from build123d import *

# Parameters (mm, degrees)
SCHIZZO1_R                    = 18
ESTRUSIONE_ESTRUSIONE1_DEPTH  = 49.54
SCHIZZO2_R                    = 2.495
ESTRUSIONE_ESTRUSIONE2_DEPTH  = 2.5
SCHIZZO3_R                    = 1.575
ESTRUSIONE_ESTRUSIONE3_DEPTH  = 12.7
SCHIZZO4_R                    = 7.67
ESTRUSIONE_ESTRUSIONE4_DEPTH  = 5
SCHIZZO5_R                    = 4.01
ESTRUSIONE_ESTRUSIONE5_DEPTH  = 9.03
FORO_FILETTATO_M3X0_5_1_D     = 2.5
FORO_FILETTATO_M3X0_5_1_DEPTH = 9
FORO_FILETTATO_M3X0_5_1_TIP   = 0.751075774
ESTRUSIONE_ESTRUSIONE6_START  = -9.1
ESTRUSIONE_ESTRUSIONE6_DEPTH  = 9.1
ESTRUSIONE_ESTRUSIONE7_START  = -4.55
ESTRUSIONE_ESTRUSIONE7_DEPTH  = 3.4


with BuildPart() as part:
    # Schizzo1 → Estrusione-Estrusione1 (new body)
    with BuildSketch(Plane(origin=(0, 0, 0), x_dir=(0, 0, -1), z_dir=(1, 0, 0))):
        Circle(SCHIZZO1_R)
    extrude(amount=ESTRUSIONE_ESTRUSIONE1_DEPTH)

    # Schizzo2 → Estrusione-Estrusione2 (add)
    with BuildSketch(Plane.ZY):
        with Locations(Location((0, 0, 0), (0, 0, 180))):
            Circle(SCHIZZO2_R)
    extrude(amount=ESTRUSIONE_ESTRUSIONE2_DEPTH)

    # Schizzo3 → Estrusione-Estrusione3 (add)
    with BuildSketch(Plane.ZY.offset(2.5)):
        Circle(SCHIZZO3_R)
    extrude(amount=ESTRUSIONE_ESTRUSIONE3_DEPTH)

    # Schizzo4 → Estrusione-Estrusione4 (add)
    with BuildSketch(Plane.ZY.offset(13.72)):
        Circle(SCHIZZO4_R)
    extrude(amount=-ESTRUSIONE_ESTRUSIONE4_DEPTH)

    # Schizzo5 → Estrusione-Estrusione5 (add)
    with BuildSketch(Plane.ZY.offset(13.72)):
        Circle(SCHIZZO5_R)
    extrude(amount=-ESTRUSIONE_ESTRUSIONE5_DEPTH)

    # Foro filettato M3x0.5-1
    with Locations(Plane.ZY):
        with Locations((12.5, 0), (6.25, -10.825317547), (-6.25, -10.825317547), (-12.5, 0), (-6.25, 10.825317547), (6.25, 10.825317547)):
            Hole(FORO_FILETTATO_M3X0_5_1_D / 2, depth=FORO_FILETTATO_M3X0_5_1_DEPTH)
            with Locations((0, 0, -(FORO_FILETTATO_M3X0_5_1_DEPTH + FORO_FILETTATO_M3X0_5_1_TIP / 2))):  # 118° drill point
                Cone(0, FORO_FILETTATO_M3X0_5_1_D / 2, FORO_FILETTATO_M3X0_5_1_TIP, mode=Mode.SUBTRACT)

    # Schizzo10 → Estrusione-Estrusione6 (add)
    with BuildSketch(Plane(origin=(49.54, 0, 0), x_dir=(0, 0, -1), z_dir=(1, 0, 0)).offset(ESTRUSIONE_ESTRUSIONE6_START)):
        with BuildLine():
            ThreePointArc((-9.925, 15.016470124), (-5.181869246, 17.237988024), (0, 18))
            Line((0, 18), (0, 19.69938782))
            ThreePointArc((0, 19.69938782), (-4.26355498, 19.232472005), (-8.325, 17.85385828))
            ThreePointArc((-8.325, 17.85385828), (-9.134600688, 17.453508265), (-9.925, 17.016470124))
            Line((-9.925, 17.016470124), (-9.925, 15.016470124))
        make_face()
        with BuildLine():
            Line((0, 19.69938782), (0, 18))
            ThreePointArc((0, 18), (5.181869246, 17.237988024), (9.925, 15.016470124))
            Line((9.925, 15.016470124), (9.925, 17.016470124))
            ThreePointArc((9.925, 17.016470124), (9.134600688, 17.453508265), (8.325, 17.85385828))
            ThreePointArc((8.325, 17.85385828), (4.26355498, 19.232472005), (0, 19.69938782))
        make_face()
    extrude(amount=ESTRUSIONE_ESTRUSIONE6_DEPTH)

    # Schizzo10<4> → Estrusione-Estrusione7 (add, symmetric)
    with BuildSketch(Plane(origin=(49.54, 0, 0), x_dir=(0, 0, -1), z_dir=(1, 0, 0)).offset(ESTRUSIONE_ESTRUSIONE7_START)):
        with BuildLine():
            ThreePointArc((-8.325, 17.85385828), (-4.26355498, 19.232472005), (0, 19.69938782))
            Line((0, 19.69938782), (0, 21.990570068))
            ThreePointArc((0, 21.990570068), (-4.24218253, 21.577512815), (-8.325, 20.35385828))
            Line((-8.325, 20.35385828), (-8.325, 17.85385828))
        make_face()
        with BuildLine():
            Line((0, 21.990570068), (0, 19.69938782))
            ThreePointArc((0, 19.69938782), (4.26355498, 19.232472005), (8.325, 17.85385828))
            Line((8.325, 17.85385828), (8.325, 20.35385828))
            ThreePointArc((8.325, 20.35385828), (4.24218253, 21.577512815), (0, 21.990570068))
        make_face()
    extrude(amount=ESTRUSIONE_ESTRUSIONE7_DEPTH, both=True)


solid = part.part
Input: part model. Units: mm. Frame: model coordinates. A direction names the side the tool comes from. Round coordinates to 2 decimals unless told otherwise and drop trailing zeros. Order: outer loops, then holes, each group sorted by start corner. A loop starts at its lowest first (then second) coordinate and runs counter-clockwise, first axis right, second up.
1. Material intervals for line 1 (Z direction, x = 7, y = 0); line 2 (Y direction, x = 6.5, z = 6.25); line 3 (Y direction, x = 3, z = 6), sorted ascending.
The answers:
line 1: z = -18 to -13.75, -11.25 to 11.25, 13.75 to 18
line 2: y = -16.88 to -12.08, -9.58 to 9.58, 12.08 to 16.88
line 3: y = -16.97 to -12.05, -9.6 to 9.6, 12.05 to 16.97
2. Cut plane A-A, the plane x = 16.5. Output: boundary loops of the cut face in (y, z).
The answers:
outline: circle Ø36 at (0, 0)
3. Pin query (flat end, axial travel): P1, Ø1, axis at x = 15, z = -9.5, coming from the -Y side; P2, Ø2.5, axis at y = 17, z = 4, coming from the -X side; P3, Ø1.5, axis at y = 8, z = -1, coming from the -X side; P4, Ø5, axis at x = 40.5, z = -1, coming from the +Y side. Return the tip coordinate at first contact, or that it passes through.
The answers:
P1: stops at y = -15.59
P2: stops at x = 0
P3: stops at x = -13.72
P4: stops at y = 21.99
4. Mould query, pull axis Y, two halves, no side actions, for faces 1 (the face through (24.423, -17.572, 3.902)), 2 (the face through (41.59, 20, 0)), 3 (the face through (9.6, -10.8, 6)). Classes: released by +Y, released by -Y, zero draft, split by the parting line, or undercut.
The answers:
face 1: split by the parting line
face 2: zero draft
face 3: undercut
5. Set-up query: faces 4 (the face through (-3.58, -0.96, -1.25)), 5 (the face through (-14.45, -0.96, -1.25)), 6 (the face through (45, 16, -9.925)), 7 (the face through (48.39, 20, 0)). Return all of +Z, -Z, +X, -X, +Y, -Y with unobstructed straight access to the full face (end or side cutting, diameter ignored); none if empty.
The answers:
face 4: none
face 5: -X
face 6: -Z, +X, -X, +Y
face 7: +X, +Y
